```python
from build123d import *

# Parameters (mm, degrees)
EKSTR_ZYON_NCE2_DEPTH = 5
RADYUS1_R             = 1


with BuildPart() as part:
    # Çizim1 → Ekstrüzyon-İnce2 (new body)
    with BuildSketch(Plane.XY):
        Polygon((148.868356189, -40.017575671), (148.868356189, -60.417575671), (128.777806905, -60.417575671), (128.777806905, -59.417575671), (147.868356189, -59.417575671), (147.868356189, -40.017575671), align=None)
    extrude(amount=EKSTR_ZYON_NCE2_DEPTH)

    # Radyus1
    radyus1_edges = [part.edges().sort_by_distance(p)[0] for p in [
        (147.868356189, -59.417575671, 2.5),
        (148.868356189, -60.417575671, 2.5),
    ]]
    fillet(radyus1_edges, radius=RADYUS1_R)


solid = part.part
```
Input: part model. Units: mm. Frame: model coordinates. A direction names the side the tool comes from. Coordinates: 2 decimals unless noted, no trailing zeros. Loops run counter-clockwise (first coordinate to the right, second up) from the corner with the lowest first, then second, coordinate; pieces in that order, holes last. Notation, with made-up numbers: (70, 0.25) - (115, 0.25) arc R28 ccw to (115, 29.25) - close; hole circle Ø5 at (-19.75, 25). An arc over 180 degrees is marked (long way). Answer in a Markdown table with one row per item.
(1) Pin query (flat end, axial travel): P1, Ø3, axis at x = 142.5, z = 4, coming from the +Y side; P2, Ø1.5, axis at y = -50, z = 2.5, coming from the -X side. Return the tip coordinate at first contact, or that it passes through.
Model answer:
| item | result |
|---|---|
| P1 | stops at y = -59.42 |
| P2 | stops at x = 147.87 |
(2) Cut plane C-C on y = -48.25. Output: boundary loops of the cut face in (x, z), plus the area to 3 significant figures.
Model answer:
| item | result |
|---|---|
| outline | (147.87, 0) - (148.87, 0) - (148.87, 5) - (147.87, 5) - close |
| area | 5.00 mm² |
(3) Cut plane A-A on z = 0.7. Output: boundary loops of the cut face in (x, y), plus the area to 3 significant figures.
Model answer:
| item | result |
|---|---|
| outline | (128.78, -60.42) - (147.87, -60.42) arc R1 ccw to (148.87, -59.42) - (148.87, -40.02) - (147.87, -40.02) - (147.87, -58.42) arc R1 cw to (146.87, -59.42) - (128.78, -59.42) - close |
| area | 39.5 mm² |
(4) Set-up query: faces 1 (the face through (148.5, -54.7, 5)), 2 (the face through (138, -59.418, 2)). Return all of +Z, -Z, +X, -X, +Y, -Y with unobstructed straight access to the full face (end or side cutting, diameter ignored); none if empty.
Model answer:
| item | result |
|---|---|
| face 1 | +Z, +X, -X, +Y, -Y |
| face 2 | +Z, -Z, -X, +Y |
(5) Material intervals for L1, parallel to Y at x = 139.5, z = 3.9; L2, parallel to X at y = -56.75, z = 0.85; L3, parallel to Y at x = 147.5, z = 1.2, sorted ascending. Write a range as from..to.
Model answer:
| item | result |
|---|---|
| L1 | y = -60.42..-59.42 |
| L2 | x = 147.87..148.87 |
| L3 | y = -60.42..-59.19 |
(6) Cut plane B-B on x = 133. Output: boundary loops of the cut face in (y, z), plus the area to 3 significant figures.
Model answer:
| item | result |
|---|---|
| outline | (-60.42, 0) - (-59.42, 0) - (-59.42, 5) - (-60.42, 5) - close |
| area | 5.00 mm² |
